Can you work these out from the model? Positions are in its coordinate system, mm. Round coordinates to 2 decimals unless told otherwise and drop trailing zeros. Order: outer loops, then holes, each group sorted by start corner. A loop starts at its lowest first (then second) coordinate and runs counter-clockwise, first axis right, second up. Notation, with made-up numbers: M 60,64.25 L 81,64.25 A18 cw 81,96.25 Z; hole C 42,25.25 d9. An arc over 180 degrees is marked long. One line per question, with ' | ' between items.
```python
from build123d import *

# Parameters (mm, degrees)
BOSS_EXTRUDE1_DEPTH = 0.7
SKETCH5_R           = 1
CUT_EXTRUDE3_DEPTH  = 5
SKETCH6_R           = 1
CUT_EXTRUDE4_DEPTH  = 6


with BuildPart() as part:
    # Sketch1 → Boss-Extrude1 (new body)
    with BuildSketch(Plane(origin=(0, 0, 0), x_dir=(1, 0, 0), z_dir=(0, 1, 0))):
        Polygon((20.240139403, -28.5), (20.75, -27.990139403), (20.75, 27.990139403), (20.240139403, 28.5), (-20.240139403, 28.5), (-20.75, 27.990139403), (-20.75, -27.990139403), (-20.240139403, -28.5), align=None)
    extrude(amount=BOSS_EXTRUDE1_DEPTH)

    # Sketch5 → Cut-Extrude3 (cut)
    with BuildSketch(Plane(origin=(0, 0.7, 0), x_dir=(1, 0, 0), z_dir=(0, 1, 0))):
        with Locations((-19, 27)):
            Circle(SKETCH5_R)
        with Locations((19, 27)):
            Circle(SKETCH5_R)
        with Locations((19, -27)):
            Circle(SKETCH5_R)
        with Locations((-19, -27)):
            Circle(SKETCH5_R)
    extrude(amount=-CUT_EXTRUDE3_DEPTH, mode=Mode.SUBTRACT)

    # Sketch6 → Cut-Extrude4 (cut)
    with BuildSketch(Plane(origin=(0, 0.7, 0), x_dir=(1, 0, 0), z_dir=(0, 1, 0))):
        with Locations((-9.45, 6.284530189)):
            Circle(SKETCH6_R)
        with Locations((-9.45, 2.115469811)):
            Circle(SKETCH6_R)
    extrude(amount=-CUT_EXTRUDE4_DEPTH, mode=Mode.SUBTRACT)


solid = part.part
```
(1) Please list where these lines run through material, in increasing order: probe 1 along X at (y, z) = (0.3, -27); probe 2 along Z at (x, y) = (-19, 0.65); probe 3 along Z at (x, y) = (-9.45, 0.55). Write a range as [from, to].
Final values:
probe 1: [-20.75, -20], [-18, 18], [20, 20.75] | probe 2: [-28.5, -28], [-26, 26], [28, 28.5] | probe 3: [-28.5, -7.28], [-5.28, -3.12], [-1.12, 28.5]
(2) Thinking about a two-plate mould opening in Z: for faces 1 (the flat face through (0, 0, 0)), 2 (the cylindrical face through (-8.526, 0.355, -1.732)), which applies, released by +Z, released by -Z, zero draft, split by the parting line, or undercut?
Final values:
face 1: zero draft | face 2: undercut
(3) If we section it at A-A on x = -9.45: Please give me the cut outline in (y, z).
Final values:
outline: M 0,-28.5 L 0.7,-28.5 L 0.7,-7.28 L 0,-7.28 Z; M 0,-5.28 L 0.7,-5.28 L 0.7,-3.12 L 0,-3.12 Z; M 0,-1.12 L 0.7,-1.12 L 0.7,28.5 L 0,28.5 Z
(4) Will these pins go through, and if not, where does the flat tip stop? pin 1 Ø1.6 at (x, z) = (-9.45, -6.28) entering from -Y; pin 2 Ø2.5 at (x, z) = (-9.45, -2.12) entering from -Y.
Final values:
pin 1: through | pin 2: y = 0
(5) If we section it at B-B on z = 27: Please give me the cut outline in (x, y), plus the area to 4 significant figures.
Final values:
outline: M -20.75,0 L -20,0 L -20,0.7 L -20.75,0.7 Z; M -18,0 L 18,0 L 18,0.7 L -18,0.7 Z; M 20,0 L 20.75,0 L 20.75,0.7 L 20,0.7 Z | area: 26.25 mm^2
